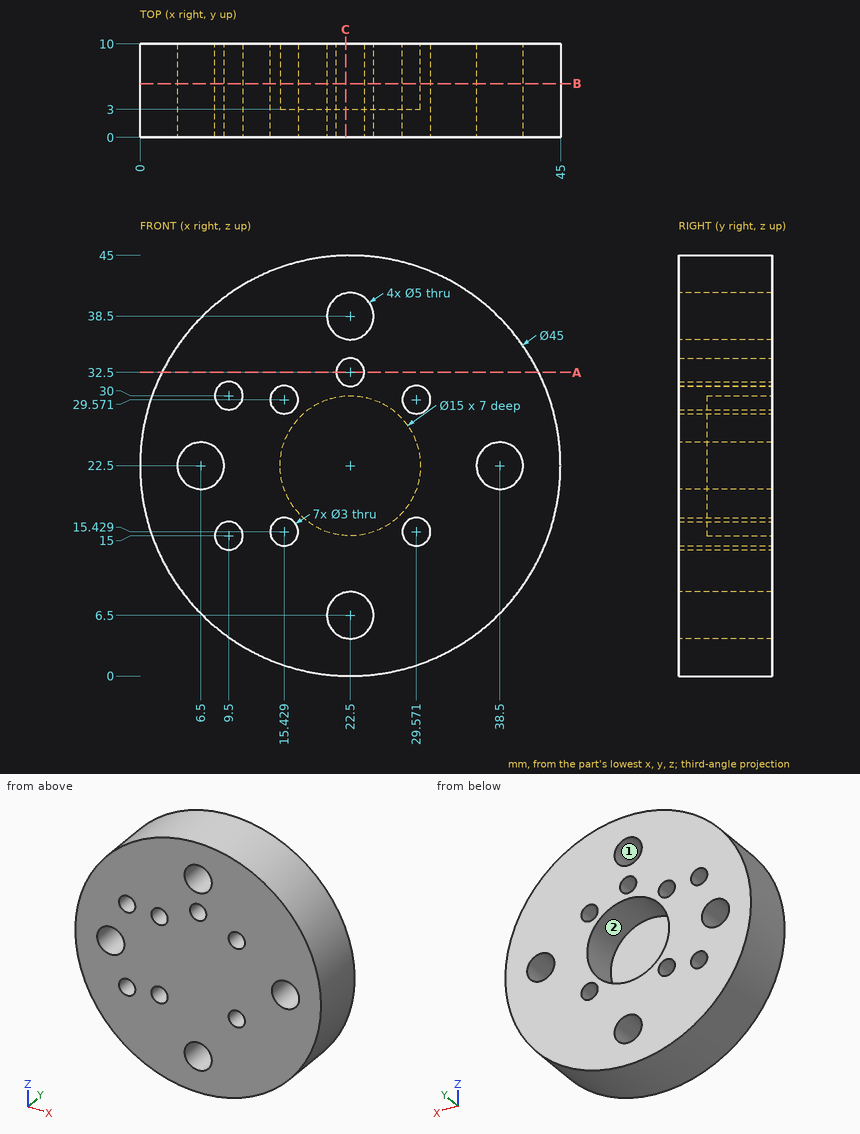
Geometry: see drawing. Coordinates: mm, zero at the bounding-box minimum. A direction names the side the tool comes from. Coordinates: 2 decimals unless noted, no trailing zeros. Order: outer loops, then holes, each group sorted by start corner. A loop starts at its lowest first (then second) coordinate and runs counter-clockwise, first axis right, second up. Notation, with made-up numbers: M -19.5,46.5 L -15.5,46.5 A15 cw -15.5,57.5 Z; hole C -6.5,-34 d3. An arc over 180 degrees is marked long. Answer in a Markdown table with one row per item. Add a question column.
Q1. Line query: L1, parallel to Z at x = 10, y = 5.5; L2, parallel to Z at x = 24.5, y = 5.5; L3, parallel to Z at x = 14.5, y = 2.5. Output: solid intervals per line, ascending.
Q2. Section query A-A on z = 32.5. Return the cut outline in (x, y), and give its area (3 significant figures).
Q3. Reachability of the marked faces 1 and 2 from +Z, -Z, +X, -X, +Y, -Y: full face, straight path, thin tool, end or side. Return the list, or none.
Q4. Section query B-B on y = 5.75. Count the separate pieces of the cut face and the enclosed holes in it, and give its area (3 significant figures).
Q5. Section query C-C on x = 22. Return the cut outline in (y, z).
Q6. Contact query for flat-ended pins moving along their axis: P1, Ø1.8, axis at x = 29.57, z = 29.57, coming from the -Y side; P2, Ø3, axis at x = 30.5, y = 6, coming from the -Z side; P3, Ø1, axis at x = 21, y = 4, coming from the -Z side; P4, Ø2, axis at y = 4, z = 17.5, coming from the +X side. Output: stop coordinate, or through.
Completed:
| question | item | result |
|---|---|---|
| 1 | L1 | z = 3.79 to 13.59, 16.41 to 28.59, 31.41 to 41.21 |
| 1 | L2 | z = 0.09 to 5, 8 to 15.27, 29.73 to 37, 40 to 44.91 |
| 1 | L3 | z = 1.47 to 14.25, 16.61 to 28.39, 30.75 to 43.53 |
| 2 | outline | M 2.34,0 L 21,0 L 21,10 L 2.34,10 Z; M 24,0 L 42.66,0 L 42.66,10 L 24,10 Z |
| 2 | area | 373 mm2 |
| 3 | face 1 | +Y, -Y |
| 3 | face 2 | +Y |
| 4 | separate pieces | 1 |
| 4 | enclosed holes | 12 |
| 4 | area | 1,290 mm2 |
| 5 | outline | M 0,0.01 L 10,0.01 L 10,4.05 L 0,4.05 Z; M 0,8.95 L 10,8.95 L 10,15.02 L 3,15.02 L 3,29.98 L 10,29.98 L 10,31.09 L 0,31.09 Z; M 0,33.91 L 10,33.91 L 10,36.05 L 0,36.05 Z; M 0,40.95 L 10,40.95 L 10,44.99 L 0,44.99 Z |
| 6 | P1 | passes through |
| 6 | P2 | stops at z = 0.96 |
| 6 | P3 | stops at z = 0.02 |
| 6 | P4 | stops at x = 44.64 |
